Autodesk Inventor part; units mm, degrees
ref_plane "YZ Plane" through (0, 0, 0) normal (1, 0, 0) x (0, 1, 0)
ref_plane "XZ Plane" through (0, 0, 0) normal (0, 1, 0) x (-1, 0, 0)
ref_plane "XY Plane" through (0, 0, 0) normal (0, 0, 1) x (1, 0, 0)
sketch "Sketch1" plane through (0, 0, 0) normal (0, 1, 0) x (-1, 0, 0)
  circle A0 centre (0, 0) radius 6.35
  circle A1 centre (0, 0) radius 3.937
  dimension "d0" = 12.7
  dimension "d1" = 7.874
extrude "Extrusion1" add sketch "Sketch1" along normal mid plane 273.05
sketch "Sketch2" plane through (0, -136.525, 0) normal (0, -1, 0) x (1, 0, 0)
  circle A0 centre (0, 0) radius 3.937
  circle A1 centre (0, 0) radius 6.35
  circle A2 centre (0, 0) radius 6.35
  line L0 (-6.35, 0) -> (0, 0)
  line L1 (6.35, 0) -> (0, 0)
  circle A3 centre (0, 0) radius 3.937
  arc A4 (3.937, 0) -> (-3.937, 0) centre (0, 0) ccw
  arc A5 (6.35, 0) -> (-6.35, 0) centre (0, 0) ccw
revolve "Revolution1" add sketch "Sketch2" angle 180 about axis through (6.35, -136.525, 0) along (1, 0, 0) picked at (-5.446, 0.8206) contours A0 L0 A1 L1
equation "\"d0\" = glassTubeDiameter"
equation "\"d1\" = glassTubeID"
equation "\"d2\" = glassTubeLength - 0.5 * glassTubeDiameter"
equation "\"tubeHeight\" = 50.8"
equation "\"tubeWidth\" = 101.6"
equation "\"tubeLength\" = 304.8"
equation "\"tubeWallThickness\" = 3.175"
equation "\"plateOverhang\" = 6.35"
equation "\"moatWidth\" = 3.175"
equation "\"moatDepth\" = 3.175"
equation "\"tubePlateClearance\" = 0.127"
equation "\"blankCapThickness\" = 9.525"
equation "\"sensorCapThickness\" = 12.7"
equation "\"glassTubeDiameter\" = 12.7"
equation "\"glassTubeClearance\" = 0.19844"
equation "\"glassTubeID\" = 7.874"
equation "\"glassTubeLength\" = 279.4"
equation "\"longHoleSpacing\" = 30.48"
equation "\"shortHoleSpacing\" = 21.59"
equation "\"sensorHolderDiameter\" = 50.8"
equation "\"sensorHolderThickness\" = 12.7"
equation "\"fiberDiameter\" = 1"
equation "\"fiberClearance\" = 0"
equation "\"oRingID\" = 22.2504"
equation "\"oRingGrooveWidth\" = 2.54"
equation "\"oRingGrooveDepth\" = 1.2446"
properties part number "glassTube" material "Glass"
For this review, take the finished solid that the model builds, in its own axes (mm). Coordinates: 2 decimals unless noted, no trailing zeros. Write each loop counter-clockwise with the first axis right and the second up, starting at its lowest first coordinate (ties: lowest second). Pieces come first, ordered by that corner, then holes. Notation, with made-up numbers: (-31, 29) - (16, 29) arc R19 cw to (16, 53) - close; hole circle Ø3 at (47.25, 62). An arc over 180 degrees is marked (long way). Answer in a Markdown table with one row per item. Add a question column.
Q1. We need section B-B, the plane z = 0. State the section outline as (x, y) points (3 decimals).
Q2. For P1, Ø1, axis at y = -33.5, z = 2.5, coming from the -X side; P2, Ø5, axis at y = -111.5, z = 3, coming from the -X side; P3, Ø4, axis at x = -4, y = 98.5, coming from the -Z side; P4, Ø4, axis at x = 0.5, z = 0, coming from the -Y side (3 decimals), all flat-tipped, find the tip position at first contact; note any pin that passes through.
Q3. We need section A-A, the plane x = 0. State the section outline as (y, z) points (3 decimals).
Q4. For probe 1 along Z at (x, y) = (0, -75.5); probe 2 along Z at (x, y) = (2.5, -40), list the stretches that pass through material, from the lowest coordinate up.
Q5. Draft analysis for pull direction Z (two halves, no side actions). For faces 1 (the cylindrical face through (0.853, -1.911, 3.843)), 2 (the flat face through (3, 136.525, -3)), 3 (the cylindrical face through (1.38, 1.91, -6.2)), state which applies: +Z half, -Z half, draft (parallel to the pull), parting line (faces both ways), or undercut.
Q6. We need section C-C, the plane y = -37.5. State the section outline as (x, z) points.
Answer list:
| question | item | result |
|---|---|---|
| 1 | outline | (-6.35, -136.525) arc R6.35 ccw to (6.35, -136.525) - (6.35, 136.525) - (3.937, 136.525) - (3.937, -136.525) arc R3.937 cw to (-3.937, -136.525) - (-3.937, 136.525) - (-6.35, 136.525) - close |
| 2 | P1 | stops at x = -6.03 |
| 2 | P2 | stops at x = -6.33 |
| 2 | P3 | stops at z = -6.03 |
| 2 | P4 | stops at y = -142.875 |
| 3 | outline | (-136.525, -6.35) - (136.525, -6.35) - (136.525, -3.937) - (-136.525, -3.937) arc R3.937 cw to (-136.525, 3.937) - (136.525, 3.937) - (136.525, 6.35) - (-136.525, 6.35) arc R6.35 ccw to start |
| 4 | probe 1 | z = -6.35 to -3.94, 3.94 to 6.35 |
| 4 | probe 2 | z = -5.84 to -3.04, 3.04 to 5.84 |
| 5 | face 1 | undercut |
| 5 | face 2 | draft |
| 5 | face 3 | parting line |
| 6 | outline | circle Ø12.7 at (0, 0); hole circle Ø7.87 at (0, 0) |
